```python
from build123d import *

# Parameters (mm, degrees)
F0_R     = 8
F0_R_2   = 5
F1_DEPTH = 11.5
F2_R     = 10
F2_R_2   = 8
F2_R_3   = 5
F3_DEPTH = 2


with BuildPart() as f1:
    # F0 (on Front) → F1 (new body, symmetric)
    with BuildSketch(Plane.XZ):
        Circle(F0_R)
        Circle(F0_R_2, mode=Mode.SUBTRACT)
    extrude(amount=F1_DEPTH, both=True)

    # F2 (on face) → F3 (join)
    with BuildSketch(Plane(origin=(0, 11.5, 0), x_dir=(-1, 0, 0), z_dir=(0, 1, 0))):
        Circle(F2_R)
        Circle(F2_R_2, mode=Mode.SUBTRACT)
        Circle(F2_R_2)
        Circle(F2_R_3, mode=Mode.SUBTRACT)
    extrude(amount=F3_DEPTH)


solid = f1.part
```
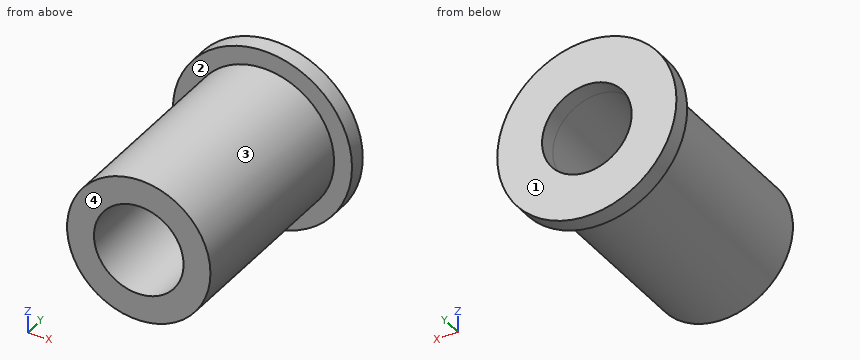
The listing builds one solid part. Answer for the finished solid, in the listing's coordinates (mm). Face numbers are marked on the shaded views. A direction names the side the tool comes from. Coordinates: 2 decimals unless noted, no trailing zeros. Write each loop counter-clockwise with the first axis right and the second up, starting at its lowest first coordinate (ties: lowest second). Pieces come first, ordered by that corner, then holes. Notation, with made-up numbers: (-7.5, 76.5) - (45.5, 76.5) arc R38 ccw to (45.5, 115.5) - close; hole circle Ø5 at (-15.5, 60). An arc over 180 degrees is marked (long way). One line per item, written item: value.
1) Find section B-B (x = 0). Give the vertices of the cut face in (y, z).
Geometry check:
outline: (-11.5, -8) - (11.5, -8) - (11.5, -10) - (13.5, -10) - (13.5, -5) - (-11.5, -5) - close; (-11.5, 5) - (13.5, 5) - (13.5, 10) - (11.5, 10) - (11.5, 8) - (-11.5, 8) - close
2) A tool of negligible diameter and unlimited length cuts with its end or side. For the marked faces 1 and 2, from which of +Z, -Z, +X, -X, +Y, -Y can it reach the whole face along a straight path? Write none if from no direction.
Geometry check:
face 1: +Z, -Z, +X, -X, +Y
face 2: -Y
3) Find section D-D (x = -5.5). Give the vertices of the cut face in (y, z), and give its area (3 significant figures).
Geometry check:
outline: (-11.5, -5.81) - (11.5, -5.81) - (11.5, -8.35) - (13.5, -8.35) - (13.5, 8.35) - (11.5, 8.35) - (11.5, 5.81) - (-11.5, 5.81) - close
area: 301 mm2
4) For a pull along X with two mould halves and no side action, classify the marked faces 3 and 4 as pulls with the +X half, pulls with the -X half, needs draft (parallel to the pull), parting line crosses it, or undercut.
Geometry check:
face 3: parting line crosses it
face 4: needs draft
5) Find section C-C (y = -6.5). Give the vertices of the cut face in (x, z), and give its area (3 significant figures).
Geometry check:
outline: circle Ø16 at (0, 0); hole circle Ø10 at (0, 0)
area: 123 mm2
6) Consider line 1 along Z through (x, y) = (0, -3.5); line 2 along Z through (x, y) = (0, 12.8); line 3 along X through (y, z) = (1, -3.5). Determine where each line is inside the solid, lowest interval first. Write a range as from..to.
Geometry check:
line 1: z = -8..-5, 5..8
line 2: z = -10..-5, 5..10
line 3: x = -7.19..-3.57, 3.57..7.19
7) Each of these flat-tipped pins is pushed along its axis until it touches: pin 1 Ø12 at (y, z) = (7, 7) entering from -X; pin 2 Ø2 at (x, z) = (3.5, 1.5) entering from -Y; pin 3 Ø6 at (x, y) = (3, 1.5) entering from +Z; pin 4 Ø10 at (x, y) = (7.5, 8.5) entering from -Z. Where does it stop, or does it pass through?
Geometry check:
pin 1: stops at x = -9.53
pin 2: passes through
pin 3: stops at z = 8
pin 4: stops at z = -9.37
8) Find section A-A (z = 0). Give the vertices of the cut face in (x, y), and give its area (3 significant figures).
Geometry check:
outline: (-10, 11.5) - (-8, 11.5) - (-8, -11.5) - (-5, -11.5) - (-5, 13.5) - (-10, 13.5) - close; (5, -11.5) - (8, -11.5) - (8, 11.5) - (10, 11.5) - (10, 13.5) - (5, 13.5) - close
area: 158 mm2
